from build123d import *

# Parameters (mm, degrees)
SKETCH_1_R      = 1.6
EXTRUDE_1_DEPTH = 3


with BuildPart() as part:
    # 草图1 → 凸台-拉伸1 (new body)
    with BuildSketch(Plane(origin=(0, 0, 0), x_dir=(1, 0, 0), z_dir=(0, 1, 0))):
        with BuildLine():
            Line((-21.134628196, 23.389975432), (-21.134628196, 18.377736005))
            ThreePointArc((-21.134628196, 18.377736005), (-21.427521415, 17.670629223), (-22.134628196, 17.377736005))
            Line((-22.134628196, 17.377736005), (-72.874730915, 17.377736005))
            ThreePointArc((-72.874730915, 17.377736005), (-73.581837696, 17.670629223), (-73.874730915, 18.377736005))
            Line((-73.874730915, 18.377736005), (-73.874730915, 23.389975432))
            ThreePointArc((-73.874730915, 23.389975432), (-74.167624134, 24.097082213), (-74.874730915, 24.389975432))
            Line((-74.874730915, 24.389975432), (-77.021723127, 24.389975432))
            ThreePointArc((-77.021723127, 24.389975432), (-79.134066788, 23.515014039), (-80.009028181, 21.402670377))
            Line((-80.009028181, 21.402670377), (-80.009028181, -28.604431477))
            ThreePointArc((-80.009028181, -28.604431477), (-79.134066788, -30.716775138), (-77.021723127, -31.591736531))
            Line((-77.021723127, -31.591736531), (-74.874730915, -31.591736531))
            ThreePointArc((-74.874730915, -31.591736531), (-74.167624134, -31.298843313), (-73.874730915, -30.591736531))
            Line((-73.874730915, -30.591736531), (-73.874730915, -25.64502865))
            ThreePointArc((-73.874730915, -25.64502865), (-73.581837696, -24.937921869), (-72.874730915, -24.64502865))
            Line((-72.874730915, -24.64502865), (-22.134628196, -24.64502865))
            ThreePointArc((-22.134628196, -24.64502865), (-21.427521415, -24.937921869), (-21.134628196, -25.64502865))
            Line((-21.134628196, -25.64502865), (-21.134628196, -30.591736531))
            ThreePointArc((-21.134628196, -30.591736531), (-20.841734977, -31.298843313), (-20.134628196, -31.591736531))
            Line((-20.134628196, -31.591736531), (12.787258331, -31.591736531))
            ThreePointArc((12.787258331, -31.591736531), (14.899601993, -30.716775138), (15.774563386, -28.604431477))
            Line((15.774563386, -28.604431477), (15.774563386, 21.402670377))
            ThreePointArc((15.774563386, 21.402670377), (14.899601993, 23.515014039), (12.787258331, 24.389975432))
            Line((12.787258331, 24.389975432), (-20.134628196, 24.389975432))
            ThreePointArc((-20.134628196, 24.389975432), (-20.841734977, 24.097082213), (-21.134628196, 23.389975432))
        make_face()
        with Locations(Location((-76.52848462, 20.886724226, 0), (0, 0, 270))):
            Circle(SKETCH_1_R, mode=Mode.SUBTRACT)
        with Locations(Location((-18.52858622, 20.886597225, 0), (0, 0, 270))):
            Circle(SKETCH_1_R, mode=Mode.SUBTRACT)
        with Locations(Location((-18.52833222, -28.113656775, 0), (0, 0, 270))):
            Circle(SKETCH_1_R, mode=Mode.SUBTRACT)
        with Locations(Location((-76.52833222, -28.113529775, 0), (0, 0, 270))):
            Circle(SKETCH_1_R, mode=Mode.SUBTRACT)
    extrude(amount=EXTRUDE_1_DEPTH)


solid = part.part
Geometry: final body of the model. Coordinates: model frame, mm. A direction names the side the tool comes from. Give positions to 0.01 mm unless a question says otherwise; leave off trailing zeros. Loops run counter-clockwise (first coordinate to the right, second up) from the corner with the lowest first, then second, coordinate; pieces in that order, holes last. Notation, with made-up numbers: M -13,-26 L 42,-26 A22 ccw 42,-9 Z; hole C -28,1.5 d5. An arc over 180 degrees is marked long. Put each result on its own line as item: value. Start each with the question number.
1) Ray query, line 1 along X through (y, z) = (2.75, -20); line 2 along Z through (x, y) = (-18, 2.35); line 3 along Z through (x, y) = (-41, 0.2). Return the intervals inside material, ascending.
2) Cut plane A-A (y = 1.55). Output: boundary loops of the cut face in (x, z), then the cut area to 3 significant figures.
3) Pull-direction query (Z, two-part tool) for faces 1 (the flat face through (-76, 1, -24.39)), 2 (the cylindrical face through (-18.458, 1.479, 26.515)), 3 (the cylindrical face through (-74.942, 1.479, -21.095)), 4 (the flat face through (-73.875, 1, 28)); classes: pulls with the +Z half, pulls with the -Z half, needs draft (parallel to the pull), parting line crosses it, or undercut.
4) Cut plane B-B (x = -67). Output: boundary loops of the cut face in (y, z).
5) Access query for faces 5 (the flat face through (-21.135, 1, -21)), 6 (the flat face through (-48, 1, 24.645)), 7 (the flat face through (-80.009, 1, 3)). Directions: +Z, -Z, +X, -X, +Y, -Y. A direction counts if a zero-diameter tool reaches every point of the face in a straight line with its end or side. Return the directions, or none.
6) Contact query for flat-ended pins moving along their axis: pin 1 (3.5 mm diameter, centred on x = -76.53, z = 28.11, fed in from -Y); pin 2 (0.9 mm diameter, centred on x = -58.5, y = 2, fed in from -Z); pin 3 (0.9 mm diameter, centred on y = 2, z = 29.5, fed in from +X). Output: stop coordinate, or through.
Verdict:
1. line 1: -80.01 to -77.86, -75.2 to -73.87, -21.13 to -19.86, -17.2 to 15.77
1. line 2: -24.39 to -22.4, -19.38 to 26.6, 29.62 to 31.59
1. line 3: -17.38 to 24.65
2. outline: M -80.01,-21.4 A2.99 ccw -77.02,-24.39 L -74.87,-24.39 A1 ccw -73.87,-23.39 L -73.87,-18.38 A1 cw -72.87,-17.38 L -22.13,-17.38 A1 cw -21.13,-18.38 L -21.13,-23.39 A1 ccw -20.13,-24.39 L 12.79,-24.39 A2.99 ccw 15.77,-21.4 L 15.77,28.6 A2.99 ccw 12.79,31.59 L -20.13,31.59 A1 ccw -21.13,30.59 L -21.13,25.65 A1 cw -22.13,24.65 L -72.87,24.65 A1 cw -73.87,25.65 L -73.87,30.59 A1 ccw -74.87,31.59 L -77.02,31.59 A2.99 ccw -80.01,28.6 Z; hole C -76.53,-20.89 d3.2; hole C -76.53,28.11 d3.2; hole C -18.53,-20.89 d3.2; hole C -18.53,28.11 d3.2
2. area: 4,590 mm2
3. face 1: pulls with the -Z half
3. face 2: undercut
3. face 3: undercut
3. face 4: needs draft
4. outline: M 0,-17.38 L 3,-17.38 L 3,24.65 L 0,24.65 Z
5. face 5: -Z, +Y, -Y
5. face 6: +Z, +Y, -Y
5. face 7: +Z, -Z, -X, +Y, -Y
6. pin 1: y = 0
6. pin 2: z = -17.38
6. pin 3: x = 15.74
